Source: three-view drawing plus pictorial views. Frame: mm from the lowest corner of the part. A direction names the side the tool comes from. Coordinates: 2 decimals unless noted, no trailing zeros. Write each loop counter-clockwise with the first axis right and the second up, starting at its lowest first coordinate (ties: lowest second). Pieces come first, ordered by that corner, then holes. Notation, with made-up numbers: (-8, -30) - (43, -30) arc R13 ccw to (43, -25) - close; hole circle Ø4 at (72.5, -8.75). An arc over 180 degrees is marked (long way). One line per item, written item: value.
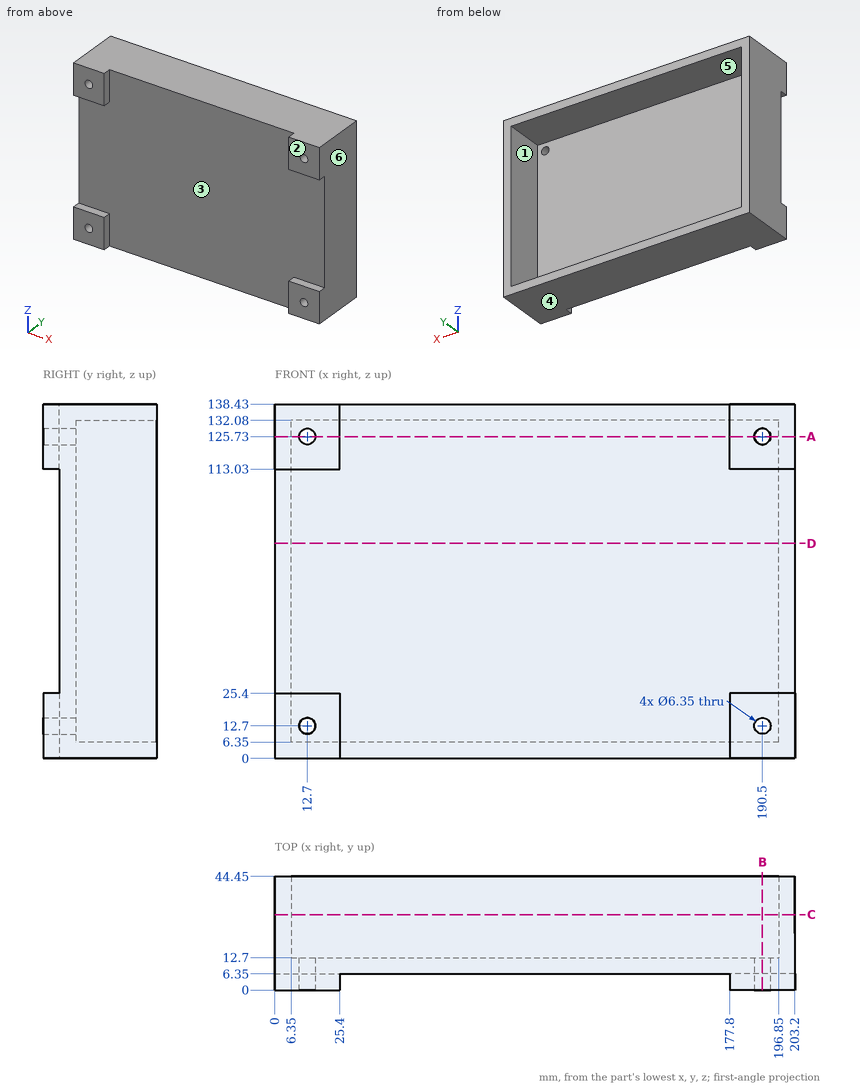
1) Draft query along Z for the marked faces 4, 5 and 6. Return one class per face: released by +Z, released by -Z, zero draft, split by the parting line, or undercut.
Values found:
face 4: released by -Z
face 5: undercut
face 6: zero draft
2) Section query C-C on y = 29.5. Output: boundary loops of the cut face in (x, z), then the cut area to 3 significant figures.
Values found:
outline: (0, 0) - (203.2, 0) - (203.2, 138.43) - (0, 138.43) - close; hole (6.35, 6.35) - (196.85, 6.35) - (196.85, 132.08) - (6.35, 132.08) - close
area: 4,180 mm2
3) Section query B-B on x = 190.5. Output: boundary loops of the cut face in (y, z) (3 decimals).
Values found:
outline: (0, 0) - (44.45, 0) - (44.45, 6.35) - (12.7, 6.35) - (12.7, 9.525) - (0, 9.525) - close; (0, 15.875) - (12.7, 15.875) - (12.7, 122.555) - (0, 122.555) - (0, 113.03) - (6.35, 113.03) - (6.35, 25.4) - (0, 25.4) - close; (0, 128.905) - (12.7, 128.905) - (12.7, 132.08) - (44.45, 132.08) - (44.45, 138.43) - (0, 138.43) - close
4) Reachability of the marked faces 1, 2 and 3 from +Z, -Z, +X, -X, +Y, -Y: full face, straight path, thin tool, end or side. Return the list, or none.
Values found:
face 1: +Y
face 2: +Z, -Z, +X, -X, -Y
face 3: -Y
5) Section query D-D on z = 84. Output: boundary loops of the cut face in (x, y).
Values found:
outline: (0, 6.35) - (203.2, 6.35) - (203.2, 44.45) - (196.85, 44.45) - (196.85, 12.7) - (6.35, 12.7) - (6.35, 44.45) - (0, 44.45) - close
6) Material intervals for line 1 (Z direction, x = 12.7, y = 3) (3 decimals); line 2 (X direction, y = 31, z = 71); line 3 (Z direction, x = 195, y = 4), sorted ascending.
Values found:
line 1: 0 to 9.525, 15.875 to 25.4, 113.03 to 122.555, 128.905 to 138.43
line 2: 0 to 6.35, 196.85 to 203.2
line 3: 0 to 25.4, 113.03 to 138.43
7) Section query A-A on z = 125.73. Output: boundary loops of the cut face in (x, y) (3 decimals), then the cut area to 3 significant figures.
Values found:
outline: (0, 0) - (9.525, 0) - (9.525, 12.7) - (6.35, 12.7) - (6.35, 44.45) - (0, 44.45) - close; (15.875, 0) - (25.4, 0) - (25.4, 6.35) - (177.8, 6.35) - (177.8, 0) - (187.325, 0) - (187.325, 12.7) - (15.875, 12.7) - close; (193.675, 0) - (203.2, 0) - (203.2, 44.45) - (196.85, 44.45) - (196.85, 12.7) - (193.675, 12.7) - close
area: 1,850 mm2
8) Contact query for flat-ended pins moving along their axis: P1, Ø10, axis at x = 176.5, z = 32, coming from the -Y side; P2, Ø8.5, axis at x = 12.7, z = 125.73, coming from the +Y side. Output: stop coordinate, or through.
Values found:
P1: y = 6.35
P2: y = 12.7
